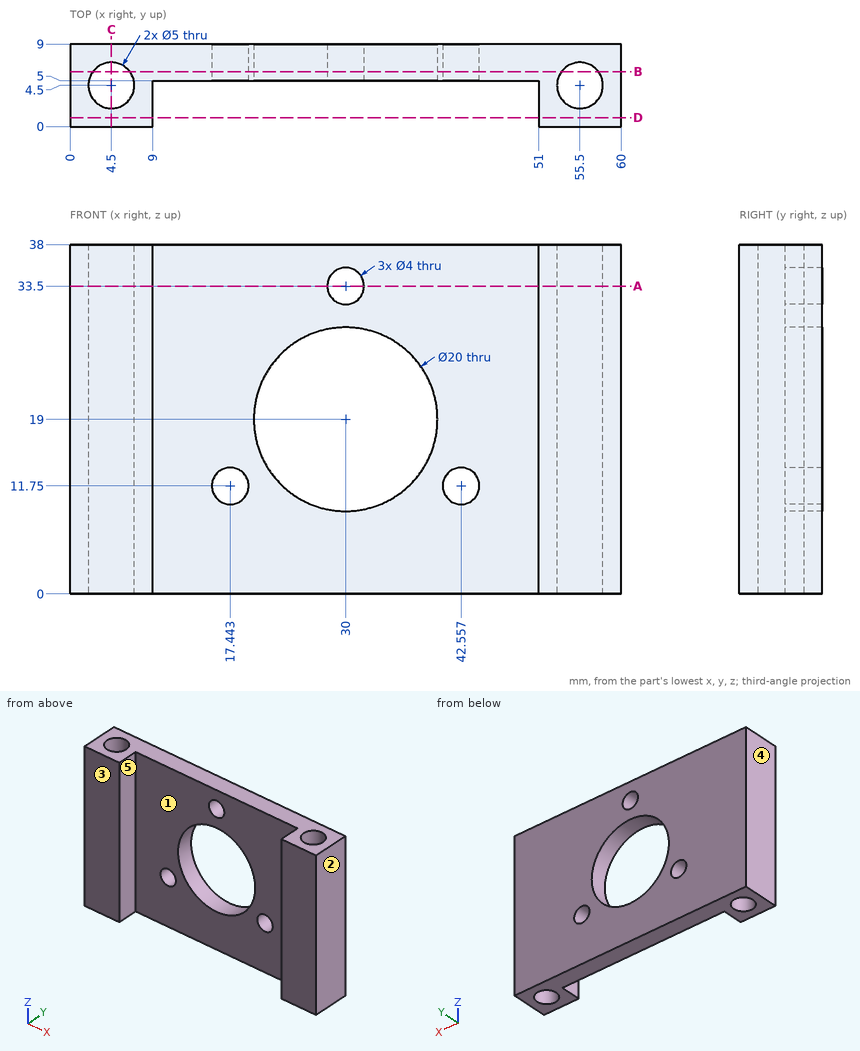
Study the drawing (mm; zero at the part's minimum x, y, z) and answer. A direction names the side the tool comes from. Round coordinates to 2 decimals unless told otherwise and drop trailing zeros. Write each loop counter-clockwise with the first axis right and the second up, starting at its lowest first coordinate (ties: lowest second). Pieces come first, ordered by that corner, then holes.
Q1. Find section C-C on x = 4.5. Determine the outline of the cut face in (y, z), and give its area (3 significant figures).
Values:
outline: (0, 0) - (2, 0) - (2, 38) - (0, 38) - close; (7, 0) - (9, 0) - (9, 38) - (7, 38) - close
area: 152 mm2
Q2. A tool of negligible diameter and unlimited length cuts with its end or side. For the marked faces 1 and 2, from which of +Z, -Z, +X, -X, +Y, -Y can it reach the whole face along a straight path? Write none if from no direction.
Values:
face 1: +Z, -Z, -Y
face 2: +Z, -Z, +X, +Y, -Y
Q3. The mould has two halves that part along X. Classify the marked faces 3, 4 and 5: released by +X, released by -X, zero draft, split by the parting line, or undercut.
Values:
face 3: zero draft
face 4: released by -X
face 5: undercut
Q4. Flat-ended cylindrical pins translate along their axes: P1, Ø12, axis at x = 30, z = 19, coming from the -Y side; P2, Ø11.5, axis at x = 26, z = 25.5, coming from the -Y side. Find the tip coordinate at first contact, or state that the pin passes through.
Values:
P1: passes through
P2: stops at y = 5
Q5. Find section A-A on z = 33.5. Determine the outline of the cut face in (x, y).
Values:
outline: (0, 0) - (9, 0) - (9, 5) - (28, 5) - (28, 9) - (0, 9) - close; (32, 5) - (51, 5) - (51, 0) - (60, 0) - (60, 9) - (32, 9) - close; hole circle Ø5 at (4.5, 4.5); hole circle Ø5 at (55.5, 4.5)
Q6. Find section B-B on y = 6. Determine the outline of the cut face in (x, z).
Values:
outline: (0, 0) - (2.5, 0) - (2.5, 38) - (0, 38) - close; (6.5, 0) - (53.5, 0) - (53.5, 38) - (6.5, 38) - close; (57.5, 0) - (60, 0) - (60, 38) - (57.5, 38) - close; hole circle Ø4 at (17.44, 11.75); hole circle Ø20 at (30, 19); hole circle Ø4 at (30, 33.5); hole circle Ø4 at (42.56, 11.75)
Q7. Find section D-D on y = 1. Determine the outline of the cut face in (x, z).
Values:
outline: (0, 0) - (9, 0) - (9, 38) - (0, 38) - close; (51, 0) - (60, 0) - (60, 38) - (51, 38) - close
Q8. Straight lines are drawn through the part: line 1 (Z direction, x = 30, y = 7.9); line 2 (Y direction, x = 55.5, z = 26); line 3 (X direction, y = 0.5, z = 24). For each, find the intervals that lie inside material, in ascending order.
Values:
line 1: z = 0 to 9, 29 to 31.5, 35.5 to 38
line 2: y = 0 to 2, 7 to 9
line 3: x = 0 to 9, 51 to 60
